For this review, take the finished solid that the model builds, in its own axes (mm). Coordinates: 2 decimals unless noted, no trailing zeros. Order: outer loops, then holes, each group sorted by start corner. A loop starts at its lowest first (then second) coordinate and runs counter-clockwise, first axis right, second up.
from build123d import *

# Parameters (mm, degrees)
SKETCH1_W         = 210
SKETCH1_H         = 210
MAINEXTRUDE_DEPTH = 4
SKETCH1_6_R       = 1.5
SCREWHOLES_DEPTH  = 4
ROUNDEDCORNERS_R  = 10
SKETCH2_R         = 2
SKETCH2_R_2       = 0.98
PCBHOLES_DEPTH    = 2
PCBROUNDS_R       = 2


with BuildPart() as part:
    # Sketch1 → MainExtrude (new body)
    with BuildSketch(Plane(origin=(0, 0, 0), x_dir=(1, 0, 0), z_dir=(0, 1, 0))):
        Rectangle(SKETCH1_W, SKETCH1_H)
    extrude(amount=MAINEXTRUDE_DEPTH)

    # Sketch1<6> → ScrewHoles (cut)
    with BuildSketch(Plane(origin=(0, 0, 0), x_dir=(1, 0, 0), z_dir=(0, 1, 0))):
        with Locations(Location((-99.833273811, 99.833273811, 0), (0, 0, 270))):
            Circle(SKETCH1_6_R)
        with Locations(Location((-99.833273811, -99.833273811, 0), (0, 0, 90))):
            Circle(SKETCH1_6_R)
        with Locations(Location((99.833273811, -99.833273811, 0), (0, 0, 270))):
            Circle(SKETCH1_6_R)
        with Locations(Location((99.833273811, 99.833273811, 0), (0, 0, 90))):
            Circle(SKETCH1_6_R)
    extrude(amount=SCREWHOLES_DEPTH, mode=Mode.SUBTRACT)

    # RoundedCorners
    roundedcorners_edges = [part.edges().sort_by_distance(p)[0] for p in [
        (-105, 2, -105),
        (-105, 2, 105),
        (105, 2, 105),
        (105, 2, -105),
    ]]
    fillet(roundedcorners_edges, radius=ROUNDEDCORNERS_R)

    # Sketch2 → PCBHoles (add)
    # profile 1 of 4: a face of its own
    with BuildSketch(Plane.XZ):
        with Locations(Location((-17.92, 37.135, 0), (0, 0, 90))):
            Circle(SKETCH2_R)
        with Locations(Location((-17.92, 37.135, 0), (0, 0, 270))):
            Circle(SKETCH2_R_2, mode=Mode.SUBTRACT)
    # profile 2 of 4: a face of its own
    with BuildSketch(Plane.XZ):
        with Locations(Location((17.92, 37.135, 0), (0, 0, 90))):
            Circle(SKETCH2_R)
        with Locations(Location((17.92, 37.135, 0), (0, 0, 270))):
            Circle(SKETCH2_R_2, mode=Mode.SUBTRACT)
    # profile 3 of 4: a face of its own
    with BuildSketch(Plane.XZ):
        with Locations(Location((-17.92, -37.135, 0), (0, 0, 90))):
            Circle(SKETCH2_R)
        with Locations(Location((-17.92, -37.135, 0), (0, 0, 90))):
            Circle(SKETCH2_R_2, mode=Mode.SUBTRACT)
    # profile 4 of 4: a face of its own
    with BuildSketch(Plane.XZ):
        with Locations(Location((17.92, -37.135, 0), (0, 0, 90))):
            Circle(SKETCH2_R)
        with Locations(Location((17.92, -37.135, 0), (0, 0, 90))):
            Circle(SKETCH2_R_2, mode=Mode.SUBTRACT)
    extrude(amount=PCBHOLES_DEPTH)

    # PCBRounds
    pcbrounds_edges = [part.edges().sort_by_distance(p)[0] for p in [
        (-17.92, 0, -39.135),
        (17.92, 0, -39.135),
        (-17.92, 0, 35.135),
        (17.92, 0, 35.135),
    ]]
    fillet(pcbrounds_edges, radius=PCBROUNDS_R - 0.0001)  # a hair under: the kernel refuses the full size


solid = part.part
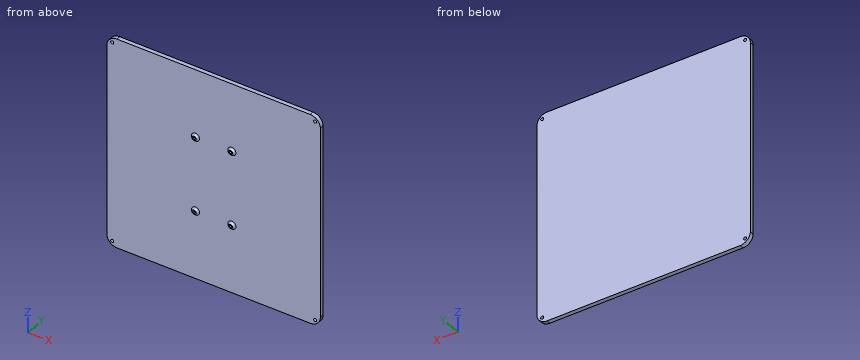
1. To check wall thickness, follow L1, parallel to Y at x = 40, z = -81; L2, parallel to X at y = -1.4, z = 36. State the ranges of each line that lie inside material, in increasing order.
Answer below:
L1: y = 0 to 4
L2: x = -19.68 to -16.16, 16.16 to 19.68
2. Clearance check with flat-ended pins moving along their axes: pin 1 Ø1.6 at (x, z) = (17.92, -37.135) entering from -Y; pin 2 Ø1.5 at (y, z) = (-1.5, 80.5) entering from -X. State where each tip first meets the part, or that it passes through.
Answer below:
pin 1: stops at y = 0
pin 2: passes through
3. Take a section at A-A, the plane x = 82. Give the boundary of the cut face in (y, z), plus the area to 3 significant figures.
Answer below:
outline: (0, -105) - (4, -105) - (4, 105) - (0, 105) - close
area: 840 mm2
4. Take a section at B-B, the plane z = -85. Give the boundary of the cut face in (x, y), plus the area to 3 significant figures.
Answer below:
outline: (-105, 0) - (105, 0) - (105, 4) - (-105, 4) - close
area: 840 mm2
